```python
from build123d import *

# Parameters (mm, degrees)
F0_W     = 127
F0_H     = 21.425162
F1_DEPTH = 25.4
F2_R     = 3.175
F3_DEPTH = 127


with BuildPart() as f1:
    # F0 (on Front) → F1 (new body)
    with BuildSketch(Plane.XZ):
        Rectangle(F0_W, F0_H)
    extrude(amount=F1_DEPTH)

    # F2 (on face) → F3 (join)
    with BuildSketch(Plane.XZ):
        with Locations((54.658038, 0)):
            Circle(F2_R)
        with Locations((-52.021962, 0)):
            Circle(F2_R)
    extrude(amount=-F3_DEPTH)


solid = f1.part
```
Part model, mm, in its own coordinate system. A direction names the side the tool comes from. Round coordinates to 2 decimals unless told otherwise and drop trailing zeros. Loops run counter-clockwise (first coordinate to the right, second up) from the corner with the lowest first, then second, coordinate; pieces in that order, holes last.
Item 1: Cut at C-C, the plane x = 2.5. Give the cut face in (y, z), then the cut area to 3 significant figures.
Item 2: Cut at D-D, the plane z = 8.5. Give the cut face in (x, y), then the cut area to 3 significant figures.
Item 3: Drop a flat-ended pin along its axis: P1, Ø12, axis at x = -19, z = 6.5, coming from the +Y side. Give the stop position or say it passes through.
Item 4: Cut at B-B, the plane y = 93. Give the cut face in (x, z) (3 decimals), then the cut area to 3 significant figures.
Item 5: Cut at A-A, the plane z = 0. Give the cut face in (x, y), then the cut area to 3 significant figures.
Item 6: 3-axis set-ups, long thin cutter, end or side, ignore diameter. For faces 4 (the face through (-48.994, 62.611, 0.954)), 5 (the face through (-63.5, -13, 0)): which of +Z, -Z, +X, -X, +Y, -Y reach the whole face in a straight line?
Item 7: Mould opens along X. For faces 1 (the face through (57.686, 62.611, 0.954)), 2 (the face through (63.5, -13, 0)), 3 (the face through (-1, -25.4, 0)) say: +X half, -X half, draft (parallel to the pull), parting line (faces both ways), or undercut.
Item 8: Drill centre lines: line 1 (X direction, y = 105, z = -0.5); line 2 (Y direction, x = -5.5, z = 1.5); line 3 (X direction, y = 74.5, z = 2.25). Where is each one in solid material? Low to high.
A:
1. outline: (-25.4, -10.71) - (0, -10.71) - (0, 10.71) - (-25.4, 10.71) - close
1. area: 544 mm2
2. outline: (-63.5, -25.4) - (63.5, -25.4) - (63.5, 0) - (-63.5, 0) - close
2. area: 3,230 mm2
3. P1: stops at y = 0
4. outline: circle Ø6.35 at (-52.022, 0); circle Ø6.35 at (54.658, 0)
4. area: 63.3 mm2
5. outline: (-63.5, -25.4) - (63.5, -25.4) - (63.5, 0) - (57.83, 0) - (57.83, 127) - (51.48, 127) - (51.48, 0) - (-48.85, 0) - (-48.85, 127) - (-55.2, 127) - (-55.2, 0) - (-63.5, 0) - close
5. area: 4,840 mm2
6. face 4: +Y
6. face 5: +Z, -Z, -X, +Y, -Y
7. face 1: undercut
7. face 2: +X half
7. face 3: draft
8. line 1: x = -55.16 to -48.89, 51.52 to 57.79
8. line 2: y = -25.4 to 0
8. line 3: x = -54.26 to -49.78, 52.42 to 56.9
